from build123d import *

# Parameters (mm, degrees)
F0_R     = 12.7
F1_DEPTH = 44.45
F2_R     = 6.35
F3_DEPTH = 12.701


with BuildPart() as f1:
    # F0 (on Front) → F1 (new body)
    with BuildSketch(Plane.XZ):
        with BuildLine():
            ThreePointArc((57.748717, 16.796402), (46.756889, 21.022344), (43.962452, 32.462187))
            ThreePointArc((43.962452, 32.462187), (42.407297, 56.789571), (21.084465, 68.603839))
            ThreePointArc((21.084465, 68.603839), (-0.238367, 56.789571), (-1.793522, 32.462187))
            ThreePointArc((-1.793522, 32.462187), (-4.587959, 21.022344), (-15.579787, 16.796402))
            Line((-15.579787, 16.796402), (-42.276816, 16.796402))
            Line((-42.276816, 16.796402), (-42.554254, 16.796402))
            Line((-42.554254, 16.796402), (-42.554254, 4.096402))
            Line((-42.554254, 4.096402), (84.445746, 4.096402))
            Line((84.445746, 4.096402), (84.445746, 16.796402))
            Line((84.445746, 16.796402), (57.748717, 16.796402))
        make_face()
        with Locations((20.945746, 43.204218)):
            Circle(F0_R, mode=Mode.SUBTRACT)
    extrude(amount=F1_DEPTH)

    # F2 (on face) → F3 (cut, through all)
    with BuildSketch(Plane.XY.offset(16.796402)):
        with Locations((65.834609, -19.05)):
            Circle(F2_R)
        with Locations((-23.504254, -19.05)):
            Circle(F2_R)
    extrude(amount=-F3_DEPTH, mode=Mode.SUBTRACT)


solid = f1.part
Check sheet for the modelled part. Datum: model origin and axes. Units: mm. A direction names the side the tool comes from. Round coordinates to 2 decimals unless told otherwise and drop trailing zeros. Loops run counter-clockwise (first coordinate to the right, second up) from the corner with the lowest first, then second, coordinate; pieces in that order, holes last. Notation, with made-up numbers: M 74,11 L 115,11 A24 ccw 115,24 Z; hole C 35.5,11 d1. An arc over 180 degrees is marked long. One line per question, with ' | ' between items. Start each with the question number.
Item 1: Section check B-B (y = -19.05). Record the boundary of the cut face in (x, z).
Item 2: Gauge pin test, flat ends, axial feed: pin 1 Ø1 at (y, z) = (-6, 46.5) entering from +X; pin 2 Ø1.5 at (y, z) = (-10.5, 23.5) entering from -X; pin 3 Ø10 at (y, z) = (-37, 38.5) entering from +X. Record the tip position at first contact, or that the pin passes through.
Item 3: Set-up check for faces 5 (the face through (10.867, -21.914, 35.476)), 6 (the face through (-32, -22, 16.796)): record each of +Z, -Z, +X, -X, +Y, -Y from which the full face is reachable in a straight line by a thin tool's end or side.
Item 4: Scan lines: probe 1 along X at (y, z) = (-19, 12); probe 2 along Z at (x, y) = (21.5, -36); probe 3 along Z at (x, y) = (78.5, -38.5). Record each from-to range of solid material in increasing order.
Item 5: Section check A-A (x = -22.5). Record the boundary of the cut face in (y, z).
Item 6: Section check D-D (z = 45.5). Record the boundary of the cut face in (x, y).
Item 7: Release check for a two-part mould opening along Z. For faces 1 (the face through (84.446, -22, 10)), 2 (the face through (74, -22, 16.796)), 3 (the face through (20, -22, 4.096)), 4 (the face through (42.596, -21.914, 56.487)) record: released by +Z, released by -Z, zero draft, split by the parting line, or undercut.
Item 8: Section check C-C (z = 11). Record the boundary of the cut face in (x, y), and give its area (3 significant figures).
Worked out:
1) outline: M -42.55,4.1 L -29.85,4.1 L -29.85,16.8 L -42.55,16.8 Z; M -17.15,4.1 L 59.48,4.1 L 59.48,16.8 L 57.75,16.8 A12.7 cw 43.96,32.46 A25.4 ccw 21.08,68.6 A25.4 ccw -1.79,32.46 A12.7 cw -15.58,16.8 L -17.15,16.8 Z; M 72.18,4.1 L 84.45,4.1 L 84.45,16.8 L 72.18,16.8 Z; hole C 20.95,43.2 d25.4
2) pin 1: x = 46.19 | pin 2: x = -3.31 | pin 3: x = 46.35
3) face 5: +Y, -Y | face 6: +Z, -X, +Y, -Y
4) probe 1: -42.55 to -29.85, -17.15 to 59.48, 72.18 to 84.45 | probe 2: 4.1 to 30.52, 55.89 to 68.6 | probe 3: 4.1 to 16.8
5) outline: M -44.45,4.1 L -25.32,4.1 L -25.32,16.8 L -44.45,16.8 Z; M -12.78,4.1 L 0,4.1 L 0,16.8 L -12.78,16.8 Z
6) outline: M -4.07,-44.45 L 8.45,-44.45 L 8.45,0 L -4.07,0 Z; M 33.44,-44.45 L 46.24,-44.45 L 46.24,0 L 33.44,0 Z
7) face 1: zero draft | face 2: released by +Z | face 3: released by -Z | face 4: undercut
8) outline: M -42.55,-44.45 L 84.45,-44.45 L 84.45,0 L -42.55,0 Z; hole C -23.5,-19.05 d12.7; hole C 65.83,-19.05 d12.7 | area: 5,390 mm^2
